CAD build for the part. Positions are in the model's coordinates, mm. A direction names the side the tool comes from. Round coordinates to 2 decimals unless told otherwise and drop trailing zeros. Write each loop counter-clockwise with the first axis right and the second up, starting at its lowest first coordinate (ties: lowest second). Pieces come first, ordered by that corner, then holes. Notation, with made-up numbers: (48.25, 19.5) -> (86.25, 19.5) arc R35 ccw to (86.25, 53.5) -> close; hole circle Ø10 at (-40, -24.5). An arc over 180 degrees is marked (long way). Answer in a Markdown table with one row per item. Add a question column.
```python
from build123d import *

# Parameters (mm, degrees)
CYLINDER010_R          = 1.6
CYLINDER010_DEPTH      = 10
CYLINDER012_R          = 1.6
CYLINDER012_DEPTH      = 10
CYLINDER011_R          = 1.6
CYLINDER011_DEPTH      = 10
CYLINDER013_R          = 1.6
CYLINDER013_DEPTH      = 10
BOX014_W               = 16
BOX014_H               = 3
BOX014_DEPTH           = 4
BOX014_PLACEMENT_ANGLE = 90
BOX018_W               = 5
BOX018_H               = 3
BOX018_DEPTH           = 3
BOX018_PLACEMENT_ANGLE = 90
BOX013_W               = 16
BOX013_H               = 3
BOX013_DEPTH           = 4
BOX013_PLACEMENT_ANGLE = 90
BOX015_W               = 25
BOX015_H               = 6
BOX015_DEPTH           = 4
BOX016_W               = 25
BOX016_H               = 6
BOX016_DEPTH           = 4
BOX017_W               = 5
BOX017_H               = 3
BOX017_DEPTH           = 3
CYLINDER004_R          = 3
CYLINDER004_DEPTH      = 2
CYLINDER005_R          = 3
CYLINDER005_DEPTH      = 2
CYLINDER008_R          = 1.6
CYLINDER008_DEPTH      = 10
CYLINDER007_R          = 1.6
CYLINDER007_DEPTH      = 10
CYLINDER009_R          = 1.6
CYLINDER009_DEPTH      = 10
CYLINDER006_R          = 1.6
CYLINDER006_DEPTH      = 10
BOX012_W               = 21
BOX012_H               = 3
BOX012_DEPTH           = 4
CYLINDER001_R          = 3
CYLINDER001_DEPTH      = 10
CYLINDER002_R          = 3
CYLINDER002_DEPTH      = 10
CYLINDER_R             = 3
CYLINDER_DEPTH         = 10
CYLINDER003_R          = 3
CYLINDER003_DEPTH      = 10
BOX011_W               = 5
BOX011_H               = 22
BOX011_DEPTH           = 10
BOX009_W               = 10
BOX009_H               = 41
BOX009_DEPTH           = 10
BOX010_W               = 10
BOX010_H               = 41
BOX010_DEPTH           = 10
BOX006_W               = 17
BOX006_H               = 13
BOX006_DEPTH           = 10
BOX_W                  = 102
BOX_H                  = 85
BOX_DEPTH              = 4


with BuildPart() as cylinder010:
    # Cylinder010 → Cylinder010 (new body)
    with BuildSketch(Plane(origin=(3.6, 5.69, 0), x_dir=(1, 0, 0), z_dir=(0, 0, 1))):
        Circle(CYLINDER010_R)
    extrude(amount=CYLINDER010_DEPTH)


with BuildPart() as cylinder012:
    # Cylinder012 → Cylinder012 (new body)
    with BuildSketch(Plane(origin=(96, 5.69, 0), x_dir=(1, 0, 0), z_dir=(0, 0, 1))):
        Circle(CYLINDER012_R)
    extrude(amount=CYLINDER012_DEPTH)


with BuildPart() as cylinder011:
    # Cylinder011 → Cylinder011 (new body)
    with BuildSketch(Plane(origin=(3.6, 82, 0), x_dir=(1, 0, 0), z_dir=(0, 0, 1))):
        Circle(CYLINDER011_R)
    extrude(amount=CYLINDER011_DEPTH)


with BuildPart() as cylinder013:
    # Cylinder013 → Cylinder013 (new body)
    with BuildSketch(Plane(origin=(96, 82, 0), x_dir=(1, 0, 0), z_dir=(0, 0, 1))):
        Circle(CYLINDER013_R)
    extrude(amount=CYLINDER013_DEPTH)


with BuildPart() as pins_sd_card_reader:
    # Box014 → Box014 (new body)
    with BuildSketch(Plane.XY):
        with Locations((8, 1.5)):
            Rectangle(BOX014_W, BOX014_H)
    extrude(amount=BOX014_DEPTH)


with BuildPart() as pins_sd_card_reader_1:
    # Box014 placement: moved
    add(pins_sd_card_reader.part.moved(Location((39, 42.5, 0))).rotate(Axis((39, 42.5, 0), (0, 0, 1)), BOX014_PLACEMENT_ANGLE))


with BuildPart() as smd_capacitor:
    # Box018 → Box018 (new body)
    with BuildSketch(Plane.XY):
        with Locations((2.5, 1.5)):
            Rectangle(BOX018_W, BOX018_H)
    extrude(amount=BOX018_DEPTH)


with BuildPart() as smd_capacitor_1:
    # Box018 placement: moved
    add(smd_capacitor.part.moved(Location((15.5, 47.5, 0))).rotate(Axis((15.5, 47.5, 0), (0, 0, 1)), BOX018_PLACEMENT_ANGLE))


with BuildPart() as pins_bluetooth:
    # Box013 → Box013 (new body)
    with BuildSketch(Plane.XY):
        with Locations((8, 1.5)):
            Rectangle(BOX013_W, BOX013_H)
    extrude(amount=BOX013_DEPTH)


with BuildPart() as pins_bluetooth_1:
    # Box013 placement: moved
    add(pins_bluetooth.part.moved(Location((92, 3.5, 0))).rotate(Axis((92, 3.5, 0), (0, 0, 1)), BOX013_PLACEMENT_ANGLE))


with BuildPart() as box015:
    # Box015 → Box015 (new body)
    with BuildSketch(Plane(origin=(29, 62, 0), x_dir=(1, 0, 0), z_dir=(0, 0, 1))):
        with Locations((12.5, 3)):
            Rectangle(BOX015_W, BOX015_H)
    extrude(amount=BOX015_DEPTH)


with BuildPart() as box016:
    # Box016 → Box016 (new body)
    with BuildSketch(Plane(origin=(29, 20, 0), x_dir=(1, 0, 0), z_dir=(0, 0, 1))):
        with Locations((12.5, 3)):
            Rectangle(BOX016_W, BOX016_H)
    extrude(amount=BOX016_DEPTH)


with BuildPart() as smd_resistor:
    # Box017 → Box017 (new body)
    with BuildSketch(Plane(origin=(11.5, 28.5, 0), x_dir=(1, 0, 0), z_dir=(0, 0, 1))):
        with Locations((2.5, 1.5)):
            Rectangle(BOX017_W, BOX017_H)
    extrude(amount=BOX017_DEPTH)


with BuildPart() as cylinder004:
    # Cylinder004 → Cylinder004 (new body)
    with BuildSketch(Plane(origin=(86.99, 68.6, 0), x_dir=(1, 0, 0), z_dir=(0, 0, 1))):
        Circle(CYLINDER004_R)
    extrude(amount=CYLINDER004_DEPTH)


with BuildPart() as cylinder005:
    # Cylinder005 → Cylinder005 (new body)
    with BuildSketch(Plane(origin=(71.83, 68.6, 0), x_dir=(1, 0, 0), z_dir=(0, 0, 1))):
        Circle(CYLINDER005_R)
    extrude(amount=CYLINDER005_DEPTH)


with BuildPart() as cylinder008:
    # Cylinder008 → Cylinder008 (new body)
    with BuildSketch(Plane(origin=(96, 5.69, 0), x_dir=(1, 0, 0), z_dir=(0, 0, 1))):
        Circle(CYLINDER008_R)
    extrude(amount=CYLINDER008_DEPTH)


with BuildPart() as cylinder007:
    # Cylinder007 → Cylinder007 (new body)
    with BuildSketch(Plane(origin=(3.6, 82, 0), x_dir=(1, 0, 0), z_dir=(0, 0, 1))):
        Circle(CYLINDER007_R)
    extrude(amount=CYLINDER007_DEPTH)


with BuildPart() as cylinder009:
    # Cylinder009 → Cylinder009 (new body)
    with BuildSketch(Plane(origin=(96, 82, 0), x_dir=(1, 0, 0), z_dir=(0, 0, 1))):
        Circle(CYLINDER009_R)
    extrude(amount=CYLINDER009_DEPTH)


with BuildPart() as board_holes:
    # Cylinder006 → Cylinder006 (new body)
    with BuildSketch(Plane(origin=(3.6, 5.69, 0), x_dir=(1, 0, 0), z_dir=(0, 0, 1))):
        Circle(CYLINDER006_R)
    extrude(amount=CYLINDER006_DEPTH)

    # Fusion004: union Cylinder008, Cylinder007, Cylinder009
    add(cylinder008.part)
    add(cylinder007.part)
    add(cylinder009.part)


with BuildPart() as obj1:
    # Box012 → Box012 (new body)
    with BuildSketch(Plane(origin=(69, 79, 0), x_dir=(1, 0, 0), z_dir=(0, 0, 1))):
        with Locations((10.5, 1.5)):
            Rectangle(BOX012_W, BOX012_H)
    extrude(amount=BOX012_DEPTH)

    # Fusion003: union pins_sd card reader, SMD capacitor, pins_bluetooth, Box015, Box016, SMD resistor, Cylinder004, Cylinder005, board holes
    add(pins_sd_card_reader_1.part)
    add(smd_capacitor_1.part)
    add(pins_bluetooth_1.part)
    add(box015.part)
    add(box016.part)
    add(smd_resistor.part)
    add(cylinder004.part)
    add(cylinder005.part)
    add(board_holes.part)

    # Fusion005: union Cylinder010, Cylinder012, Cylinder011, Cylinder013
    add(cylinder010.part)
    add(cylinder012.part)
    add(cylinder011.part)
    add(cylinder013.part)


with BuildPart() as cylinder001:
    # Cylinder001 → Cylinder001 (new body)
    with BuildSketch(Plane(origin=(26.3, 63.91, 0), x_dir=(1, 0, 0), z_dir=(0, 0, 1))):
        Circle(CYLINDER001_R)
    extrude(amount=CYLINDER001_DEPTH)


with BuildPart() as cylinder002:
    # Cylinder002 → Cylinder002 (new body)
    with BuildSketch(Plane(origin=(65.19, 23.81, 0), x_dir=(1, 0, 0), z_dir=(0, 0, 1))):
        Circle(CYLINDER002_R)
    extrude(amount=CYLINDER002_DEPTH)


with BuildPart() as cylinder:
    # Cylinder → Cylinder (new body)
    with BuildSketch(Plane(origin=(26.3, 23.81, 0), x_dir=(1, 0, 0), z_dir=(0, 0, 1))):
        Circle(CYLINDER_R)
    extrude(amount=CYLINDER_DEPTH)


with BuildPart() as cylinder003:
    # Cylinder003 → Cylinder003 (new body)
    with BuildSketch(Plane(origin=(65.19, 63.91, 0), x_dir=(1, 0, 0), z_dir=(0, 0, 1))):
        Circle(CYLINDER003_R)
    extrude(amount=CYLINDER003_DEPTH)


with BuildPart() as screen_holes:
    # Box011 → Box011 (new body)
    with BuildSketch(Plane(origin=(24, 33, 0), x_dir=(1, 0, 0), z_dir=(0, 0, 1))):
        with Locations((2.5, 11)):
            Rectangle(BOX011_W, BOX011_H)
    extrude(amount=BOX011_DEPTH)

    # Fusion002: union Cylinder001, Cylinder002, Cylinder, Cylinder003
    add(cylinder001.part)
    add(cylinder002.part)
    add(cylinder.part)
    add(cylinder003.part)


with BuildPart() as button_array:
    # Box009 → Box009 (new body)
    with BuildSketch(Plane(origin=(70.5, 23, 0), x_dir=(1, 0, 0), z_dir=(0, 0, 1))):
        with Locations((5, 20.5)):
            Rectangle(BOX009_W, BOX009_H)
    extrude(amount=BOX009_DEPTH)


with BuildPart() as button_arrays:
    # Box010 → Box010 (new body)
    with BuildSketch(Plane(origin=(85.5, 23, 0), x_dir=(1, 0, 0), z_dir=(0, 0, 1))):
        with Locations((5, 20.5)):
            Rectangle(BOX010_W, BOX010_H)
    extrude(amount=BOX010_DEPTH)

    # Fusion001: union button array
    add(button_array.part)


with BuildPart() as led_array_connector:
    # Box006 → Box006 (new body)
    with BuildSketch(Plane(origin=(-11, 20.5, 0), x_dir=(1, 0, 0), z_dir=(0, 0, 1))):
        with Locations((8.5, 6.5)):
            Rectangle(BOX006_W, BOX006_H)
    extrude(amount=BOX006_DEPTH)


with BuildPart() as final_top:
    # Box → Box (new body)
    with BuildSketch(Plane(origin=(-2, 0, 1), x_dir=(1, 0, 0), z_dir=(0, 0, 1))):
        with Locations((51, 42.5)):
            Rectangle(BOX_W, BOX_H)
    extrude(amount=BOX_DEPTH)

    # Cut001: cut led array connector
    add(led_array_connector.part, mode=Mode.SUBTRACT)

    # Cut002: cut button arrays
    add(button_arrays.part, mode=Mode.SUBTRACT)

    # Cut003: cut screen holes
    add(screen_holes.part, mode=Mode.SUBTRACT)

    # Cut004: cut obj1
    add(obj1.part, mode=Mode.SUBTRACT)


solid = final_top.part
```
Item 1: Drill centre lines: probe 1 along X at (y, z) = (44.5, 2.4); probe 2 along X at (y, z) = (68.6, 1.55); probe 3 along Y at (x, z) = (26.3, 3.5). Where is each one in solid material? Low to high.
Item 2: Two-plate mould, pull along X, no slides. Class faces 1 (the flat face through (48, 85, 3)), 2 (the flat face through (14, 31.5, 2)), 3 (the flat face through (26, 55, 3)), 4 (the flat face through (100, 42, 3)): +X half, -X half, draft (parallel to the pull), parting line (faces both ways), or undercut.
Item 3: Saw through at A-A on x = 26.3. Give the cut face in (y, z).
Item 4: Saw through at C-C on x = 65.19. Give the cut face in (y, z).
Item 5: Saw through at B-B on y = 37.5. Give the cut face in (x, z), then the cut area to 3 significant figures.
Item 6: Pin check, flat tip, straight feed: pin 1 (1.8 mm diameter, centred on x = 41, y = 23.5, fed in from -Z). Stop position of the tip, or through.
Item 7: Tool access for faces 5 (the flat face through (11.5, 30, 2)), 6 (the flat face through (48, 43, 5)), 7 (the flat face through (29, 44, 3)): list every direction of +Z, -Z, +X, -X, +Y, -Y with a clear straight run to the whole face (end or side of a thin tool).
Recorded:
| question | item | result |
|---|---|---|
| 1 | probe 1 | -2 to 24, 29 to 36, 39 to 70.5, 80.5 to 85.5, 95.5 to 100 |
| 1 | probe 2 | -2 to 68.83, 74.83 to 83.99, 89.99 to 100 |
| 1 | probe 3 | 0 to 20.81, 26.81 to 33, 55 to 60.91, 66.91 to 85 |
| 2 | face 1 | draft |
| 2 | face 2 | undercut |
| 2 | face 3 | undercut |
| 2 | face 4 | +X half |
| 3 | outline | (0, 1) -> (20.81, 1) -> (20.81, 5) -> (0, 5) -> close; (26.81, 1) -> (33, 1) -> (33, 5) -> (26.81, 5) -> close; (55, 1) -> (60.91, 1) -> (60.91, 5) -> (55, 5) -> close; (66.91, 1) -> (85, 1) -> (85, 5) -> (66.91, 5) -> close |
| 4 | outline | (0, 1) -> (20.81, 1) -> (20.81, 5) -> (0, 5) -> close; (26.81, 1) -> (60.91, 1) -> (60.91, 5) -> (26.81, 5) -> close; (66.91, 1) -> (85, 1) -> (85, 5) -> (66.91, 5) -> close |
| 5 | outline | (-2, 1) -> (24, 1) -> (24, 5) -> (-2, 5) -> close; (29, 1) -> (70.5, 1) -> (70.5, 5) -> (29, 5) -> close; (80.5, 1) -> (85.5, 1) -> (85.5, 5) -> (80.5, 5) -> close; (95.5, 1) -> (100, 1) -> (100, 5) -> (95.5, 5) -> close |
| 5 | area | 308 mm2 |
| 6 | pin 1 | z = 4 |
| 7 | face 5 | -Z |
| 7 | face 6 | +Z, +X, -X, +Y, -Y |
| 7 | face 7 | +Z, -Z |
